Check sheet for the modelled part. Datum: model origin and axes. Units: mm. Coordinates: 2 decimals unless noted, no trailing zeros. Loops run counter-clockwise (first coordinate to the right, second up) from the corner with the lowest first, then second, coordinate; pieces in that order, holes last.
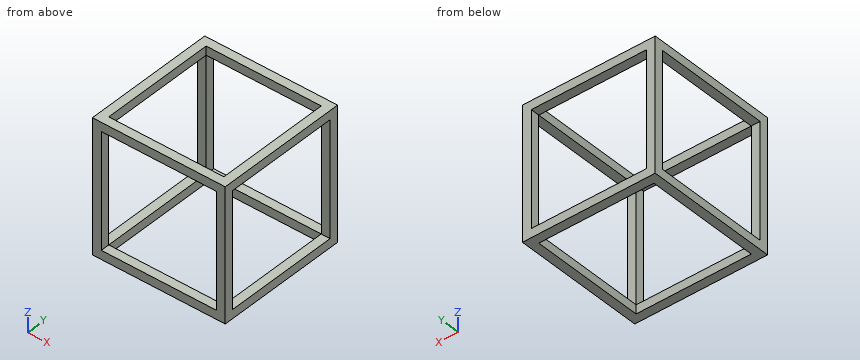
```python
from build123d import *

# Parameters (mm, degrees)
F0_W     = 30
F0_H     = 30
F1_DEPTH = 30
F2_W     = 26
F2_H     = 26
F3_DEPTH = 30.001
F4_W     = 26
F4_H     = 26
F5_DEPTH = 30.001
F6_W     = 26
F6_H     = 26
F7_DEPTH = 30.001


with BuildPart() as f1:
    # F0 (on Right) → F1 (new body)
    with BuildSketch(Plane.YZ):
        with Locations((15, 15)):
            Rectangle(F0_W, F0_H)
    extrude(amount=F1_DEPTH)

    # F2 (on face) → F3 (cut, through all)
    with BuildSketch(Plane.XZ):
        with Locations((15, 15)):
            Rectangle(F2_W, F2_H)
    extrude(amount=-F3_DEPTH, mode=Mode.SUBTRACT)

    # F4 (on face) → F5 (cut, through all)
    with BuildSketch(Plane(origin=(0, 0, 0), x_dir=(0, -1, 0), z_dir=(-1, 0, 0))):
        with Locations((-15, 15)):
            Rectangle(F4_W, F4_H)
    extrude(amount=-F5_DEPTH, mode=Mode.SUBTRACT)

    # F6 (on face) → F7 (cut, through all)
    with BuildSketch(Plane.XY.offset(30)):
        with Locations((15, 15)):
            Rectangle(F6_W, F6_H)
    extrude(amount=-F7_DEPTH, mode=Mode.SUBTRACT)


solid = f1.part
```
1) Scan line: line 1 (X direction, y = 4.25, z = 28.75). Record every from-to range of solid material in increasing order.
Answer sheet:
line 1: x = 0 to 2, 28 to 30
2) Section check A-A on x = 9.5. Enter the section's corners in (y, z).
Answer sheet:
outline: (0, 0) - (2, 0) - (2, 2) - (0, 2) - close; (0, 28) - (2, 28) - (2, 30) - (0, 30) - close; (28, 0) - (30, 0) - (30, 2) - (28, 2) - close; (28, 28) - (30, 28) - (30, 30) - (28, 30) - close
